Input: part model. Units: mm. Frame: model coordinates. A direction names the side the tool comes from. Give positions to 0.01 mm unless a question says otherwise; leave off trailing zeros. Write each loop counter-clockwise with the first axis right and the second up, starting at its lowest first coordinate (ties: lowest second). Pieces come first, ordered by that corner, then holes. Notation, with made-up numbers: (75.25, 38) - (104.25, 38) arc R32 cw to (104.25, 68) - close; hole circle Ø6 at (20, 59). An arc over 180 degrees is marked (long way). Answer as CSV lines item,"result". Start each with the question number.
from build123d import *

# Parameters (mm, degrees)
SKETCH_1_R      = 1
SKETCH_1_W      = 80.34314575
SKETCH_1_H      = 52.34314575
EXTRUDE_1_DEPTH = 3
FILLET_1_R      = 2


with BuildPart() as part:
    # 草图1 → 凸台-拉伸1 (new body)
    with BuildSketch(Plane.XY):
        with BuildLine():
            Line((2.828427125, 60.828427125), (83.171572875, 60.828427125))
            ThreePointArc((83.171572875, 60.828427125), (88.828427125, 60.828427125), (88.828427125, 55.171572875))
            Line((88.828427125, 55.171572875), (88.828427125, 2.828427125))
            ThreePointArc((88.828427125, 2.828427125), (88.828427125, -2.828427125), (83.171572875, -2.828427125))
            Line((83.171572875, -2.828427125), (2.828427125, -2.828427125))
            ThreePointArc((2.828427125, -2.828427125), (-2.828427125, -2.828427125), (-2.828427125, 2.828427125))
            Line((-2.828427125, 2.828427125), (-2.828427125, 55.171572875))
            ThreePointArc((-2.828427125, 55.171572875), (-2.828427125, 60.828427125), (2.828427125, 60.828427125))
        make_face()
        with Locations((0, 58)):
            Circle(SKETCH_1_R, mode=Mode.SUBTRACT)
        Circle(SKETCH_1_R, mode=Mode.SUBTRACT)
        with Locations((86, 58)):
            Circle(SKETCH_1_R, mode=Mode.SUBTRACT)
        with Locations((86, 0)):
            Circle(SKETCH_1_R, mode=Mode.SUBTRACT)
        with Locations((43, 29)):
            Rectangle(SKETCH_1_W, SKETCH_1_H, mode=Mode.SUBTRACT)
    extrude(amount=EXTRUDE_1_DEPTH)

    # 圆角1
    fillet_1_edges = [part.edges().sort_by_distance(p)[0] for p in [
        (83.171572875, 2.828427125, 1.5),
        (83.171572875, 55.171572875, 1.5),
        (2.828427125, 55.171572875, 1.5),
        (2.828427125, 2.828427125, 1.5),
    ]]
    fillet(fillet_1_edges, radius=FILLET_1_R)


solid = part.part
1) Material intervals for line 1 (Y direction, x = 86, z = 2.3); line 2 (Y direction, x = 64.5, z = 2.2); line 3 (X direction, y = 6, z = 2), sorted ascending. Write a range as from..to.
2) Reachability of faces 4 (the flat face through (44, 0, 0)), 5 (the flat face through (-2.828, 29, 1)), 6 (the cylindrical face through (82.6, 3.43, 1.52)) from +Z, -Z, +X, -X, +Y, -Y: full face, straight path, thin tool, end or side. Return the list, or none.
3) Cut plane B-B on y = 58. Output: boundary loops of the cut face in (x, z), and give its area (3 significant figures).
4) Pull-direction query (Y, two-part tool) for faces 1 (the flat face through (42, 60.828, 1)), 2 (the cylindrical face through (-2.89, 60.766, 1.479)), 3 (the flat face through (44, -2.828, 1)); classes: +Y half, -Y half, draft (parallel to the pull), parting line (faces both ways), or undercut.
5) Cut plane C-C on x = 0. Output: boundary loops of the cut face in (y, z), and give its area (3 significant figures).
6) Contact query for flat-ended pins moving along their axis: P1, Ø1.5, axis at x = 18, z = 1, coming from the -Y side; P2, Ø10, axis at x = 6.5, y = 51.5, coming from the -Z side; P3, Ø1.5, axis at x = 33.5, z = 2, coming from the +Y side; P4, Ø0.9, axis at y = 37.5, z = 1, coming from the -X side. Output: stop coordinate, or through.
7) Cut plane D-D on z = 1. Output: boundary loops of the cut face in (x, y).
8) Cut plane A-A on x = 72.5. Output: boundary loops of the cut face in (y, z), and give its area (3 significant figures).
Numbers:
1,line 1,"y = -4..-1, 1..57, 59..62"
1,line 2,"y = -2.83..2.83, 55.17..60.83"
1,line 3,"x = -2.83..2.83, 83.17..88.83"
2,face 4,"-Z, +X, -X, +Y, -Y"
2,face 5,"+Z, -Z, -X"
2,face 6,"+Z, -Z"
3,outline,"(-4, 0) - (-1, 0) - (-1, 3) - (-4, 3) - close; (1, 0) - (85, 0) - (85, 3) - (1, 3) - close; (87, 0) - (90, 0) - (90, 3) - (87, 3) - close"
3,area,"270 mm²"
4,face 1,"+Y half"
4,face 2,"undercut"
4,face 3,"-Y half"
5,outline,"(-4, 0) - (-1, 0) - (-1, 3) - (-4, 3) - close; (1, 0) - (57, 0) - (57, 3) - (1, 3) - close; (59, 0) - (62, 0) - (62, 3) - (59, 3) - close"
5,area,"186 mm²"
6,P1,"stops at y = -2.83"
6,P2,"stops at z = 0"
6,P3,"stops at y = 60.83"
6,P4,"stops at x = -2.83"
7,outline,"(-2.83, 2.83) arc R4 ccw to (2.83, -2.83) - (83.17, -2.83) arc R4 ccw to (88.83, 2.83) - (88.83, 55.17) arc R4 ccw to (83.17, 60.83) - (2.83, 60.83) arc R4 ccw to (-2.83, 55.17) - close; hole circle Ø2 at (0, 0); hole circle Ø2 at (0, 58); hole (2.83, 4.83) arc R2 ccw to (4.83, 2.83) - (81.17, 2.83) arc R2 ccw to (83.17, 4.83) - (83.17, 53.17) arc R2 ccw to (81.17, 55.17) - (4.83, 55.17) arc R2 ccw to (2.83, 53.17) - close; hole circle Ø2 at (86, 0); hole circle Ø2 at (86, 58)"
8,outline,"(-2.83, 0) - (2.83, 0) - (2.83, 3) - (-2.83, 3) - close; (55.17, 0) - (60.83, 0) - (60.83, 3) - (55.17, 3) - close"
8,area,"33.9 mm²"
